Geometry: final body of the model. Coordinates: model frame, mm. Face numbers are marked on the shaded views. A direction names the side the tool comes from. Give positions to 0.01 mm unless a question says otherwise; leave off trailing zeros. Order: outer loops, then holes, each group sorted by start corner. A loop starts at its lowest first (then second) coordinate and runs counter-clockwise, first axis right, second up. Notation, with made-up numbers: (55.5, -29) -> (96.5, -29) arc R19 ccw to (96.5, -25) -> close; hole circle Ø11 at (11, 29). An arc over 180 degrees is marked (long way). One line per question, with ' | ' between items.
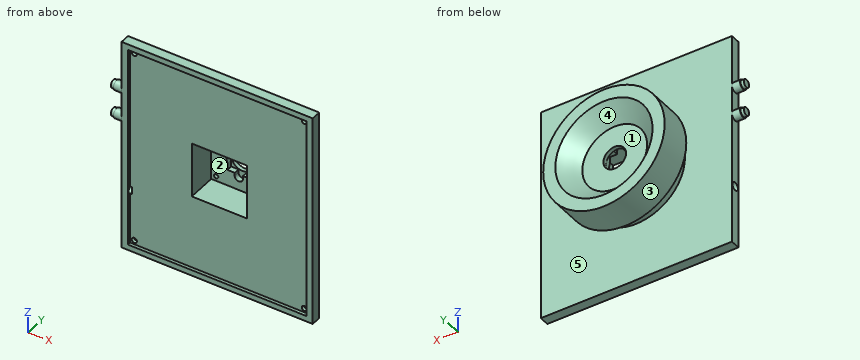
from build123d import *

# Parameters (mm, degrees)
SKETCH_1_W          = 118
SKETCH_1_H          = 132
EXTRUDE_1_DEPTH     = 6
SKETCH_2_W          = 110
SKETCH_2_H          = 125
CUT_EXTRUDE_1_DEPTH = 2
SKETCH_3_R          = 30
EXTRUDE_2_DEPTH     = 10
SKETCH_4_R          = 37.5
EXTRUDE_3_DEPTH     = 20
SKETCH_6_R          = 20
SKETCH_7_R          = 30
SKETCH_8_R          = 1.6
CUT_EXTRUDE_2_DEPTH = 2.2
SKETCH_10_W         = 34
SKETCH_10_H         = 34
CUT_EXTRUDE_3_DEPTH = 18
CUT_EXTRUDE_4_DEPTH = 3.5
SKETCH_12_R         = 7
CUT_EXTRUDE_5_DEPTH = 93.265920036
SKETCH_13_R         = 1.35
CUT_EXTRUDE_6_DEPTH = 2
SKETCH_14_R         = 3
EXTRUDE_4_DEPTH     = 5
SKETCH_15_R         = 2.5
EXTRUDE_5_DEPTH     = 2
SKETCH_16_R         = 2.5
CUT_EXTRUDE_7_DEPTH = 5


with BuildPart() as part:
    # 草图1 → 凸台-拉伸1 (new body)
    with BuildSketch(Plane(origin=(0, 0, 0), x_dir=(1, 0, 0), z_dir=(0, 1, 0))):
        Rectangle(SKETCH_1_W, SKETCH_1_H)
    extrude(amount=EXTRUDE_1_DEPTH)

    # 草图2 → 切除-拉伸1 (cut)
    with BuildSketch(Plane.XZ):
        Rectangle(SKETCH_2_W, SKETCH_2_H)
    extrude(amount=-CUT_EXTRUDE_1_DEPTH, mode=Mode.SUBTRACT)

    # 草图3 → 凸台-拉伸2 (add)
    with BuildSketch(Plane(origin=(0, 6, 0), x_dir=(1, 0, 0), z_dir=(0, 1, 0))):
        with Locations(Location((0, 0, 0), (0, 0, 270))):
            Circle(SKETCH_3_R)
    extrude(amount=EXTRUDE_2_DEPTH)

    # 草图4 → 凸台-拉伸3 (add)
    with BuildSketch(Plane(origin=(0, 16, 0), x_dir=(1, 0, 0), z_dir=(0, 1, 0))):
        with Locations(Location((0, 0, 0), (0, 0, 270))):
            Circle(SKETCH_4_R)
    extrude(amount=EXTRUDE_3_DEPTH)

    # 草图6 → 切除-放样2 section 0
    with BuildSketch(Plane(origin=(0, 26, 0), x_dir=(1, 0, 0), z_dir=(0, 1, 0))):
        Circle(SKETCH_6_R)
    # 草图7 → 切除-放样2 section 1
    with BuildSketch(Plane(origin=(0, 36, 0), x_dir=(1, 0, 0), z_dir=(0, 1, 0))):
        Circle(SKETCH_7_R)
    loft(mode=Mode.SUBTRACT)

    # 草图8 → 切除-拉伸2 (cut)
    with BuildSketch(Plane.XZ.offset(-2)):
        with Locations(Location((52.5, 60, 0), (0, 0, 270))):
            Circle(SKETCH_8_R)
        with Locations(Location((52.5, -60, 0), (0, 0, 270))):
            Circle(SKETCH_8_R)
        with Locations(Location((-52.5, -60, 0), (0, 0, 270))):
            Circle(SKETCH_8_R)
        with Locations(Location((-52.5, 60, 0), (0, 0, 270))):
            Circle(SKETCH_8_R)
    extrude(amount=-CUT_EXTRUDE_2_DEPTH, mode=Mode.SUBTRACT)

    # 草图10 → 切除-拉伸3 (cut)
    with BuildSketch(Plane.XZ.offset(-2)):
        Rectangle(SKETCH_10_W, SKETCH_10_H)
    extrude(amount=-CUT_EXTRUDE_3_DEPTH, mode=Mode.SUBTRACT)

    # 草图11 → 切除-拉伸4 (cut)
    with BuildSketch(Plane.XZ.offset(-20)):
        with BuildLine():
            Line((-2.687978229, -7), (-7, -7))
            Line((-7, -7), (-7, -2.690813124))
            ThreePointArc((-7, -2.690813124), (-7.5, 0.001769279), (-7, 2.694351683))
            Line((-7, 2.694351683), (-7, 7))
            Line((-7, 7), (-2.697177558, 7))
            ThreePointArc((-2.697177558, 7), (-2.598843965, 7.03710936), (-2.5, 7.072837091))
            Line((-2.5, 7.072837091), (-2.5, 9.133061324))
            ThreePointArc((-2.5, 9.133061324), (0, 11.503538559), (2.5, 9.133061324))
            Line((2.5, 9.133061324), (2.5, 7.072837091))
            ThreePointArc((2.5, 7.072837091), (2.598843965, 7.03710936), (2.697177558, 7))
            Line((2.697177558, 7), (7, 7))
            Line((7, 7), (7, 2.694351683))
            ThreePointArc((7, 2.694351683), (7.5, 0.001769279), (7, -2.690813124))
            Line((7, -2.690813124), (7, -7))
            Line((7, -7), (2.687978229, -7))
            ThreePointArc((2.687978229, -7), (2.594220518, -7.035276969), (2.5, -7.069298532))
            Line((2.5, -7.069298532), (2.5, -9))
            ThreePointArc((2.5, -9), (0, -11.5), (-2.5, -9))
            Line((-2.5, -9), (-2.5, -7.069298532))
            ThreePointArc((-2.5, -7.069298532), (-2.594220518, -7.035276969), (-2.687978229, -7))
        make_face()
    extrude(amount=-CUT_EXTRUDE_4_DEPTH, mode=Mode.SUBTRACT)

    # 草图12 → 切除-拉伸5 (cut, through all)
    with BuildSketch(Plane(origin=(0, 26, 0), x_dir=(1, 0, 0), z_dir=(0, 1, 0))):
        with Locations(Location((0, 0, 0), (0, 0, 270))):
            Circle(SKETCH_12_R)
    extrude(amount=-CUT_EXTRUDE_5_DEPTH, mode=Mode.SUBTRACT)

    # 草图13 → 切除-拉伸6 (cut)
    with BuildSketch(Plane.XZ.offset(-20)):
        with Locations(Location((-14, 14, 0), (0, 0, 270))):
            Circle(SKETCH_13_R)
        with Locations(Location((14, 14, 0), (0, 0, 270))):
            Circle(SKETCH_13_R)
        with Locations(Location((14, -14, 0), (0, 0, 270))):
            Circle(SKETCH_13_R)
        with Locations(Location((-14, -14, 0), (0, 0, 270))):
            Circle(SKETCH_13_R)
    extrude(amount=-CUT_EXTRUDE_6_DEPTH, mode=Mode.SUBTRACT)

    # 草图14 → 凸台-拉伸4 (add)
    with BuildSketch(Plane.ZY.offset(59)):
        with Locations(Location((34.5, 3, 0), (0, 0, 270))):
            Circle(SKETCH_14_R)
        with Locations(Location((16.5, 3, 0), (0, 0, 270))):
            Circle(SKETCH_14_R)
    extrude(amount=EXTRUDE_4_DEPTH)

    # 草图15 → 凸台-拉伸5 (add)
    with BuildSketch(Plane.ZY.offset(64)):
        with Locations((16.5, 3)):
            Circle(SKETCH_15_R)
        with Locations((34.5, 3)):
            Circle(SKETCH_15_R)
    extrude(amount=EXTRUDE_5_DEPTH)

    # 草图16 → 切除-拉伸7 (cut)
    with BuildSketch(Plane.ZY.offset(59)):
        with Locations((-28.664816868, 3)):
            Circle(SKETCH_16_R)
    extrude(amount=-CUT_EXTRUDE_7_DEPTH, mode=Mode.SUBTRACT)


solid = part.part
1) Pull-direction query (X, two-part tool) for the marked faces 3, 4 and 5; classes: +X half, -X half, draft (parallel to the pull), parting line (faces both ways), or undercut.
Check result:
face 3: parting line | face 4: undercut | face 5: draft
2) Section A-A on y = 13. Return loops of the section in (x, z).
Check result:
outline: circle Ø60 at (0, 0); hole (-17, -17) -> (17, -17) -> (17, 17) -> (-17, 17) -> close
3) Material intervals for probe 1 along X at (y, z) = (25, 0); probe 2 along Y at (x, z) = (7.5, 32); probe 3 along Y at (x, z) = (-43, 23.5), sorted ascending. Write a range as from..to.
Check result:
probe 1: x = -37.5..-7, 7..37.5 | probe 2: y = 2..6, 16..36 | probe 3: y = 2..6
4) Set-up query: the marked faces 1 and 2. Return all of +Z, -Z, +X, -X, +Y, -Y with unobstructed straight access to the full face (end or side cutting, diameter ignored); none if empty.
Check result:
face 1: +Y | face 2: -Y
5) Section B-B on x = -49. Return loops of the section in (y, z).
Check result:
outline: (0, -66) -> (6, -66) -> (6, 66) -> (0, 66) -> (0, 62.5) -> (2, 62.5) -> (2, -62.5) -> (0, -62.5) -> close
6) Section D-D on y = 34. Return loops of the section in (x, z), plus the area to 3 significant figures.
Check result:
outline: circle Ø75 at (0, 0); hole circle Ø56 at (0, 0) | area: 1,950 mm^2
7) Contact query for flat-ended pins moving along their axis: pin 1 Ø3 at (x, y) = (-6, 21.5) entering from +Z; pin 2 Ø3 at (x, z) = (2, -15) entering from -Y; pin 3 Ø10 at (x, z) = (-40, -15.5) entering from +Y. Output: stop coordinate, or through.
Check result:
pin 1: stops at z = 37.23 | pin 2: stops at y = 20 | pin 3: stops at y = 6
8) Section C-C on z = -52. Return loops of the section in (x, y).
Check result:
outline: (-59, 0) -> (-55, 0) -> (-55, 2) -> (55, 2) -> (55, 0) -> (59, 0) -> (59, 6) -> (-59, 6) -> close
